```python
from build123d import *

# Parameters (mm, degrees)
SKETCH1_R           = 500
BOSS_EXTRUDE1_DEPTH = 600
SKETCH2_OUTSIDE_W   = 1309.246
SKETCH2_OUTSIDE_H   = 1309.246
SKETCH2_OUTSIDE_R   = 5
CUT_EXTRUDE1_DEPTH  = 29
SKETCH3_OUTSIDE_W   = 1309.246
SKETCH3_OUTSIDE_H   = 1309.246
SKETCH3_OUTSIDE_R   = 6.25
CUT_EXTRUDE2_DEPTH  = 5
SKETCH4_OUTSIDE_W   = 1309.246
SKETCH4_OUTSIDE_H   = 1309.246
SKETCH4_OUTSIDE_R   = 5.75
CUT_EXTRUDE3_DEPTH  = 1
SKETCH5_OUTSIDE_W   = 1309.246
SKETCH5_OUTSIDE_H   = 1309.246
SKETCH5_OUTSIDE_R   = 7.5
CUT_EXTRUDE4_DEPTH  = 100
SKETCH6_OUTSIDE_W   = 1309.246
SKETCH6_OUTSIDE_H   = 1309.246
SKETCH6_OUTSIDE_R   = 12.5
CUT_EXTRUDE5_DEPTH  = 300
SKETCH7_OUTSIDE_W   = 1309.246
SKETCH7_OUTSIDE_H   = 1309.246
SKETCH7_OUTSIDE_R   = 15
CUT_EXTRUDE6_DEPTH  = 25
SKETCH8_OUTSIDE_W   = 1309.246
SKETCH8_OUTSIDE_H   = 1309.246
SKETCH8_OUTSIDE_R   = 10
CUT_EXTRUDE7_DEPTH  = 100
SKETCH9_OUTSIDE_W   = 1309.246
SKETCH9_OUTSIDE_H   = 1309.246
SKETCH9_OUTSIDE_R   = 9.5
CUT_EXTRUDE8_DEPTH  = 1
SKETCH10_OUTSIDE_W  = 1309.246
SKETCH10_OUTSIDE_H  = 1309.246
SKETCH10_OUTSIDE_R  = 10
CUT_EXTRUDE10_DEPTH = 39
CUT_EXTRUDE11_DEPTH = 25


with BuildPart() as part:
    # Sketch1 → Boss-Extrude1 (new body)
    with BuildSketch(Plane(origin=(0, 0, 0), x_dir=(0, 0, -1), z_dir=(1, 0, 0))):
        Circle(SKETCH1_R)
    extrude(amount=BOSS_EXTRUDE1_DEPTH)

    # Sketch2 outside → Cut-Extrude1 (cut)
    with BuildSketch(Plane.ZY):
        Rectangle(SKETCH2_OUTSIDE_W, SKETCH2_OUTSIDE_H)
        Circle(SKETCH2_OUTSIDE_R, mode=Mode.SUBTRACT)
    extrude(amount=-CUT_EXTRUDE1_DEPTH, mode=Mode.SUBTRACT)

    # Sketch3 outside → Cut-Extrude2 (cut)
    with BuildSketch(Plane.ZY.offset(-29)):
        Rectangle(SKETCH3_OUTSIDE_W, SKETCH3_OUTSIDE_H)
        Circle(SKETCH3_OUTSIDE_R, mode=Mode.SUBTRACT)
    extrude(amount=-CUT_EXTRUDE2_DEPTH, mode=Mode.SUBTRACT)

    # Sketch4 outside → Cut-Extrude3 (cut)
    with BuildSketch(Plane.ZY.offset(-34)):
        Rectangle(SKETCH4_OUTSIDE_W, SKETCH4_OUTSIDE_H)
        Circle(SKETCH4_OUTSIDE_R, mode=Mode.SUBTRACT)
    extrude(amount=-CUT_EXTRUDE3_DEPTH, mode=Mode.SUBTRACT)

    # Sketch5 outside → Cut-Extrude4 (cut)
    with BuildSketch(Plane.ZY.offset(-35)):
        Rectangle(SKETCH5_OUTSIDE_W, SKETCH5_OUTSIDE_H)
        Circle(SKETCH5_OUTSIDE_R, mode=Mode.SUBTRACT)
    extrude(amount=-CUT_EXTRUDE4_DEPTH, mode=Mode.SUBTRACT)

    # Sketch6 outside → Cut-Extrude5 (cut)
    with BuildSketch(Plane.ZY.offset(-135)):
        Rectangle(SKETCH6_OUTSIDE_W, SKETCH6_OUTSIDE_H)
        Circle(SKETCH6_OUTSIDE_R, mode=Mode.SUBTRACT)
    extrude(amount=-CUT_EXTRUDE5_DEPTH, mode=Mode.SUBTRACT)

    # Sketch7 outside → Cut-Extrude6 (cut)
    with BuildSketch(Plane.ZY.offset(-435)):
        Rectangle(SKETCH7_OUTSIDE_W, SKETCH7_OUTSIDE_H)
        Circle(SKETCH7_OUTSIDE_R, mode=Mode.SUBTRACT)
    extrude(amount=-CUT_EXTRUDE6_DEPTH, mode=Mode.SUBTRACT)

    # Sketch8 outside → Cut-Extrude7 (cut)
    with BuildSketch(Plane.ZY.offset(-460)):
        Rectangle(SKETCH8_OUTSIDE_W, SKETCH8_OUTSIDE_H)
        Circle(SKETCH8_OUTSIDE_R, mode=Mode.SUBTRACT)
    extrude(amount=-CUT_EXTRUDE7_DEPTH, mode=Mode.SUBTRACT)

    # Sketch9 outside → Cut-Extrude8 (cut)
    with BuildSketch(Plane.ZY.offset(-560)):
        Rectangle(SKETCH9_OUTSIDE_W, SKETCH9_OUTSIDE_H)
        Circle(SKETCH9_OUTSIDE_R, mode=Mode.SUBTRACT)
    extrude(amount=-CUT_EXTRUDE8_DEPTH, mode=Mode.SUBTRACT)

    # Sketch10 outside → Cut-Extrude10 (cut)
    with BuildSketch(Plane.ZY.offset(-561)):
        Rectangle(SKETCH10_OUTSIDE_W, SKETCH10_OUTSIDE_H)
        Circle(SKETCH10_OUTSIDE_R, mode=Mode.SUBTRACT)
    extrude(amount=-CUT_EXTRUDE10_DEPTH, mode=Mode.SUBTRACT)

    # Sketch14<3> → Cut-Extrude11 (cut)
    with BuildSketch(Plane(origin=(0, 30, 0), x_dir=(1, 0, 0), z_dir=(0, 1, 0))):
        with BuildLine():
            Line((18.890286749, 1.405946281), (24.942306626, 1.405946281))
            ThreePointArc((24.942306626, 1.405946281), (26.348252906, 0), (24.942306626, -1.405946281))
            Line((24.942306626, -1.405946281), (18.890286749, -1.405946281))
            ThreePointArc((18.890286749, -1.405946281), (17.484340469, 0), (18.890286749, 1.405946281))
        make_face()
        with BuildLine():
            Line((523.62027087, 2.365533558), (532.010381059, 2.365533558))
            ThreePointArc((532.010381059, 2.365533558), (534.375914617, 0), (532.010381059, -2.365533558))
            Line((532.010381059, -2.365533558), (523.62027087, -2.365533558))
            ThreePointArc((523.62027087, -2.365533558), (521.254737312, 0), (523.62027087, 2.365533558))
        make_face()
    extrude(amount=-CUT_EXTRUDE11_DEPTH, mode=Mode.SUBTRACT)


solid = part.part
```
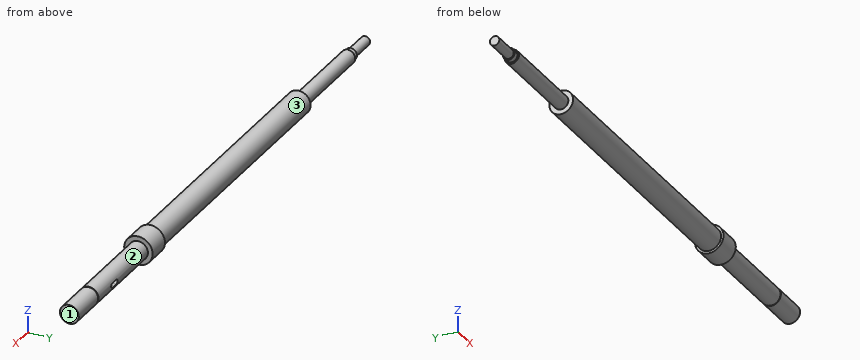
Can you work these out from the model? Positions are in its coordinate system, mm. Face numbers are marked on the shaded views. A direction names the side the tool comes from. Round coordinates to 2 decimals unless told otherwise and drop trailing zeros. Loops run counter-clockwise (first coordinate to the right, second up) from the corner with the lowest first, then second, coordinate; pieces in that order, holes last. Notation, with made-up numbers: M 7,31 L 63,31 A9 ccw 63,40 Z; hole C 65.5,-25.75 d2. An arc over 180 degrees is marked long. Answer as a JSON object with one key per item and string values. Group by question number.
Q1. Imagine slicing it at A-A, the plane x = 360. Please give me the cut outline in (y, z).
Q2. Please list where these lines run through material, in increasing order: L1, parallel to X at y = 8.75, z = 4.5; L2, parallel to X at y = 13.25, z = 1.25; L3, parallel to X at y = 10, z = -2.75.
Q3. On a 3-axis mill with a long thin cutter (end or side, diameter ignored), from which of +Z, -Z, +X, -X, +Y, -Y can I reach the whole of each face in a straight line? I mean the marked faces 1, 2 and 3. Say none if no direction works.
Q4. Will these pins go through, and if not, where does the flat tip stop? pin 1 (1.4 mm diameter, centred on x = 530, z = -0.5, fed in from +Y); pin 2 (8 mm diameter, centred on x = 287.5, y = -11, fed in from -Z); pin 3 (1 mm diameter, centred on x = 412.5, z = 7.5, fed in from -Y).
Findings:
{
 "1": {"outline": "C 0,0 d25"},
 "2": {"L1": "x = 135 to 560, 561 to 600", "L2": "x = 435 to 460", "L3": "x = 135 to 460"},
 "3": {"face 1": "+Z, -Z, +X, +Y, -Y", "face 2": "+X", "face 3": "-X"},
 "4": {"pin 1": "stops at y = 5", "pin 2": "stops at z = -10.36", "pin 3": "stops at y = -10.36"}
}
